from build123d import *

# Parameters (mm, degrees)
SKETCH1_W            = 180
SKETCH1_H            = 160
BOSS_EXTRUDE1_DEPTH  = 3
BOSS_EXTRUDE2_DEPTH  = 10
M3_CLEARANCE_HOLE1_D = 3.4


with BuildPart() as part:
    # Sketch1 → Boss-Extrude1 (new body)
    with BuildSketch(Plane(origin=(0, 0, 0), x_dir=(1, 0, 0), z_dir=(0, 1, 0))):
        Rectangle(SKETCH1_W, SKETCH1_H)
        with BuildLine():
            Line((-80, -58.195), (-76, -58.195))
            ThreePointArc((-76, -58.195), (-74.445, -59.75), (-76, -61.305))
            Line((-76, -61.305), (-80, -61.305))
            ThreePointArc((-80, -61.305), (-81.555, -59.75), (-80, -58.195))
        make_face(mode=Mode.SUBTRACT)
        with BuildLine():
            Line((-58, -58.195), (-54, -58.195))
            ThreePointArc((-54, -58.195), (-52.445, -59.75), (-54, -61.305))
            Line((-54, -61.305), (-58, -61.305))
            ThreePointArc((-58, -61.305), (-59.555, -59.75), (-58, -58.195))
        make_face(mode=Mode.SUBTRACT)
        with BuildLine():
            Line((-80, -71.695), (-76, -71.695))
            ThreePointArc((-76, -71.695), (-74.445, -73.25), (-76, -74.805))
            Line((-76, -74.805), (-80, -74.805))
            ThreePointArc((-80, -74.805), (-81.555, -73.25), (-80, -71.695))
        make_face(mode=Mode.SUBTRACT)
        with BuildLine():
            Line((-58, -71.695), (-54, -71.695))
            ThreePointArc((-54, -71.695), (-52.445, -73.25), (-54, -74.805))
            Line((-54, -74.805), (-58, -74.805))
            ThreePointArc((-58, -74.805), (-59.555, -73.25), (-58, -71.695))
        make_face(mode=Mode.SUBTRACT)
        with BuildLine():
            Line((-80, 71.695), (-76, 71.695))
            ThreePointArc((-76, 71.695), (-74.445, 73.25), (-76, 74.805))
            Line((-76, 74.805), (-80, 74.805))
            ThreePointArc((-80, 74.805), (-81.555, 73.25), (-80, 71.695))
        make_face(mode=Mode.SUBTRACT)
        with BuildLine():
            Line((-58, 71.695), (-54, 71.695))
            ThreePointArc((-54, 71.695), (-52.445, 73.25), (-54, 74.805))
            Line((-54, 74.805), (-58, 74.805))
            ThreePointArc((-58, 74.805), (-59.555, 73.25), (-58, 71.695))
        make_face(mode=Mode.SUBTRACT)
        with BuildLine():
            Line((-58, 58.195), (-54, 58.195))
            ThreePointArc((-54, 58.195), (-52.445, 59.75), (-54, 61.305))
            Line((-54, 61.305), (-58, 61.305))
            ThreePointArc((-58, 61.305), (-59.555, 59.75), (-58, 58.195))
        make_face(mode=Mode.SUBTRACT)
        with BuildLine():
            Line((-80, 58.195), (-76, 58.195))
            ThreePointArc((-76, 58.195), (-74.445, 59.75), (-76, 61.305))
            Line((-76, 61.305), (-80, 61.305))
            ThreePointArc((-80, 61.305), (-81.555, 59.75), (-80, 58.195))
        make_face(mode=Mode.SUBTRACT)
        with BuildLine():
            Line((80, -71.695), (76, -71.695))
            ThreePointArc((76, -71.695), (74.445, -73.25), (76, -74.805))
            Line((76, -74.805), (80, -74.805))
            ThreePointArc((80, -74.805), (81.555, -73.25), (80, -71.695))
        make_face(mode=Mode.SUBTRACT)
        with BuildLine():
            Line((80, -58.195), (76, -58.195))
            ThreePointArc((76, -58.195), (74.445, -59.75), (76, -61.305))
            Line((76, -61.305), (80, -61.305))
            ThreePointArc((80, -61.305), (81.555, -59.75), (80, -58.195))
        make_face(mode=Mode.SUBTRACT)
        with BuildLine():
            Line((58, -58.195), (54, -58.195))
            ThreePointArc((54, -58.195), (52.445, -59.75), (54, -61.305))
            Line((54, -61.305), (58, -61.305))
            ThreePointArc((58, -61.305), (59.555, -59.75), (58, -58.195))
        make_face(mode=Mode.SUBTRACT)
        with BuildLine():
            Line((58, -71.695), (54, -71.695))
            ThreePointArc((54, -71.695), (52.445, -73.25), (54, -74.805))
            Line((54, -74.805), (58, -74.805))
            ThreePointArc((58, -74.805), (59.555, -73.25), (58, -71.695))
        make_face(mode=Mode.SUBTRACT)
        with BuildLine():
            Line((80, 58.195), (76, 58.195))
            ThreePointArc((76, 58.195), (74.445, 59.75), (76, 61.305))
            Line((76, 61.305), (80, 61.305))
            ThreePointArc((80, 61.305), (81.555, 59.75), (80, 58.195))
        make_face(mode=Mode.SUBTRACT)
        with BuildLine():
            Line((58, 58.195), (54, 58.195))
            ThreePointArc((54, 58.195), (52.445, 59.75), (54, 61.305))
            Line((54, 61.305), (58, 61.305))
            ThreePointArc((58, 61.305), (59.555, 59.75), (58, 58.195))
        make_face(mode=Mode.SUBTRACT)
        with BuildLine():
            Line((58, 71.695), (54, 71.695))
            ThreePointArc((54, 71.695), (52.445, 73.25), (54, 74.805))
            Line((54, 74.805), (58, 74.805))
            ThreePointArc((58, 74.805), (59.555, 73.25), (58, 71.695))
        make_face(mode=Mode.SUBTRACT)
        with BuildLine():
            Line((80, 71.695), (76, 71.695))
            ThreePointArc((76, 71.695), (74.445, 73.25), (76, 74.805))
            Line((76, 74.805), (80, 74.805))
            ThreePointArc((80, 74.805), (81.555, 73.25), (80, 71.695))
        make_face(mode=Mode.SUBTRACT)
        with BuildLine():
            Line((-84, -43), (-84, 43))
            ThreePointArc((-84, 43), (-78, 49), (-72, 43))
            Line((-72, 43), (-72, -43))
            ThreePointArc((-72, -43), (-78, -49), (-84, -43))
        make_face(mode=Mode.SUBTRACT)
        with BuildLine():
            Line((77, -43), (77, 43))
            ThreePointArc((77, 43), (82, 48), (87, 43))
            Line((87, 43), (87, -43))
            ThreePointArc((87, -43), (82, -48), (77, -43))
        make_face(mode=Mode.SUBTRACT)
        with BuildLine():
            Line((-44, 60), (44, 60))
            ThreePointArc((44, 60), (49, 55), (44, 50))
            Line((44, 50), (-44, 50))
            ThreePointArc((-44, 50), (-49, 55), (-44, 60))
        make_face(mode=Mode.SUBTRACT)
        with BuildLine():
            Line((-44, -60), (44, -60))
            ThreePointArc((44, -60), (49, -55), (44, -50))
            Line((44, -50), (-44, -50))
            ThreePointArc((-44, -50), (-49, -55), (-44, -60))
        make_face(mode=Mode.SUBTRACT)
    extrude(amount=BOSS_EXTRUDE1_DEPTH)

    # Sketch1<3> → Boss-Extrude2 (add)
    with BuildSketch(Plane(origin=(0, 0, 0), x_dir=(1, 0, 0), z_dir=(0, 1, 0))):
        Polygon((-70, 47), (-70, 43), (70, 43), (70, -43), (-70, -43), (-70, -47), (74, -47), (74, 47), align=None)
    extrude(amount=BOSS_EXTRUDE2_DEPTH)

    # M3 Clearance Hole1 (through all)
    with Locations(Plane(origin=(0, 3, 0), x_dir=(1, 0, 0), z_dir=(0, 1, 0))):
        with Locations((-44, -66.5), (-34.222222222, -66.5), (-24.444444444, -66.5), (-14.666666667, -66.5), (-4.888888889, -66.5), (4.888888889, -66.5), (14.666666667, -66.5), (24.444444444, -66.5), (34.222222222, -66.5), (44, -66.5), (44, 66.5), (34.222222222, 66.5), (24.444444444, 66.5), (14.666666667, 66.5), (4.888888889, 66.5), (-4.888888889, 66.5), (-14.666666667, 66.5), (-24.444444444, 66.5), (-34.222222222, 66.5), (-44.881291433, 66.5)):
            Hole(M3_CLEARANCE_HOLE1_D / 2)


solid = part.part
Design review of the part built by this model. Coordinates are the model's own, in mm. A direction names the side the tool comes from. Round coordinates to 2 decimals unless told otherwise and drop trailing zeros. Write each loop counter-clockwise with the first axis right and the second up, starting at its lowest first coordinate (ties: lowest second). Pieces come first, ordered by that corner, then holes. Notation, with made-up numbers: M -18.75,67.5 L 19.25,67.5 A24 cw 19.25,104.5 Z; hole C 86,-38.75 d11. An arc over 180 degrees is marked long. One line per item, written item: value. Start each with the question number.
1. To check wall thickness, follow probe 1 along X at (y, z) = (0.5, -8); probe 2 along Z at (x, y) = (-17, 7.25); probe 3 along Z at (x, y) = (72, 4.75). State the ranges of each line that lie inside material, in increasing order. Write a range as from..to.
2. Take a section at A-A on x = -78. State the section outline as (y, z) points (3 decimals).
3. Take a section at B-B on z = 17.5. State the section outline as (x, y) points, then the cut area to 3 significant figures.
4. Draft analysis for pull direction X (two halves, no side actions). For faces 6 (the face through (-1, 3, -1)), 7 (the face through (49, 1, -55)), 8 (the face through (70, 6, -1)), 9 (the face through (49, 1, 55)), state which applies: pulls with the +X half, pulls with the -X half, needs draft (parallel to the pull), parting line crosses it, or undercut.
5. Clearance check with flat-ended pins moving along their axes: P1, Ø2, axis at x = 54, y = 5.5, coming from the -Z side; P2, Ø4, axis at x = 1, y = 8, coming from the +Z side; P3, Ø2, axis at x = -4.89, z = -66.5, coming from the -Y side; P4, Ø2, axis at y = 5, z = 15, coming from the +X side. State where each tip first meets the part, or that it passes through.
6. Take a section at C-C on z = 55. State the section outline as (x, y) points.
7. Take a section at D-D on y = 8. State the section outline as (x, z) points.
8. For faces 1 (the face through (-70, 6, -45)), 2 (the face through (-49, 1, -55)), 3 (the face through (-1, 6, -43)), 4 (the face through (3, 6, -47)), 5 (the face through (74, 6, 1)), list the 3-axis set-ups (+Z, -Z, +X, -X, +Y, -Y) from which the entire face can be reached by the end or side of a thin tool; tool diameter is ignored.
Computed:
1. probe 1: x = -90..-84, -72..77, 87..90
1. probe 2: z = -47..-43, 43..47
1. probe 3: z = -47..47
2. outline: M 0,-80 L 3,-80 L 3,-74.805 L 0,-74.805 Z; M 0,-71.695 L 3,-71.695 L 3,-61.305 L 0,-61.305 Z; M 0,-58.195 L 3,-58.195 L 3,-49 L 0,-49 Z; M 0,49 L 3,49 L 3,58.195 L 0,58.195 Z; M 0,61.305 L 3,61.305 L 3,71.695 L 0,71.695 Z; M 0,74.805 L 3,74.805 L 3,80 L 0,80 Z
3. outline: M -90,0 L -84,0 L -84,3 L -90,3 Z; M -72,0 L 77,0 L 77,3 L 74,3 L 74,10 L 70,10 L 70,3 L -72,3 Z; M 87,0 L 90,0 L 90,3 L 87,3 Z
3. area: 502 mm²
4. face 6: needs draft
4. face 7: undercut
4. face 8: pulls with the -X half
4. face 9: undercut
5. P1: stops at z = -47
5. P2: stops at z = 47
5. P3: passes through
5. P4: stops at x = 74
6. outline: M -90,0 L -49,0 L -49,3 L -90,3 Z; M 49,0 L 90,0 L 90,3 L 49,3 Z
7. outline: M -70,-47 L 74,-47 L 74,47 L -70,47 L -70,43 L 70,43 L 70,-43 L -70,-43 Z
8. face 1: +Z, -Z, -X, +Y
8. face 2: +Y, -Y
8. face 3: -X, +Y
8. face 4: -Z, +X, -X, +Y
8. face 5: +Z, -Z, +X, +Y
